from build123d import *

# Parameters (mm, degrees)
SKETCH1_W                = 60.014675034
SKETCH1_H                = 30.010951808
BOSS_EXTRUDE3_DEPTH      = 2
SKETCH5_R                = 0.958101179
SKETCH5_R_2              = 1
CUT_EXTRUDE2_DEPTH       = 2
BOSS_EXTRUDE5_DEPTH      = 10
BOSS_EXTRUDE5_DEPTH_BACK = 10


with BuildPart() as part:
    # Sketch1 → Boss-Extrude3 (new body)
    with BuildSketch(Plane(origin=(0, 0, 0), x_dir=(1, 0, 0), z_dir=(0, 1, 0))):
        Rectangle(SKETCH1_W, SKETCH1_H)
    extrude(amount=BOSS_EXTRUDE3_DEPTH)

    # Sketch5 → Cut-Extrude2 (cut)
    with BuildSketch(Plane(origin=(0, 2, 0), x_dir=(1, 0, 0), z_dir=(0, 1, 0))):
        with Locations(Location((28.355534017, 0, 0), (0, 0, 270))):
            Circle(SKETCH5_R)
        with Locations(Location((-28.355534017, 0, 0), (0, 0, 270))):
            Circle(SKETCH5_R_2)
    extrude(amount=-CUT_EXTRUDE2_DEPTH, mode=Mode.SUBTRACT)

    # Sketch7 → Boss-Extrude5 (add, two sides: drawn at the far end of the back side and taken through both)
    with BuildSketch(Plane.XY.offset(-BOSS_EXTRUDE5_DEPTH_BACK)):
        Polygon((7.498773608, 0), (8.961948947, 0), (8.961948947, -3.176146278), (21.045388571, -3.176146278), (21.045388571, 0), (22.508563909, 0), (22.508563909, -4.517390338), (7.498773608, -4.517390338), align=None)
        Polygon((-7.498773608, 0), (-7.498773608, -4.517390338), (-22.508563909, -4.517390338), (-22.508563909, 0), (-21.045388571, 0), (-21.045388571, -3.176146278), (-8.961948947, -3.176146278), (-8.961948947, 0), align=None)
    extrude(amount=BOSS_EXTRUDE5_DEPTH + BOSS_EXTRUDE5_DEPTH_BACK)


solid = part.part
Model file for the job. Use its own axes, mm. A direction names the side the tool comes from. Give positions to 0.01 mm unless a question says otherwise; leave off trailing zeros. Loops run counter-clockwise (first coordinate to the right, second up) from the corner with the lowest first, then second, coordinate; pieces in that order, holes last.
Item 1: Slice it at B-B (x = 17.5). Write the cut outline in (y, z), plus the area to 3 significant figures.
Check values:
outline: (-4.52, -10) - (-3.18, -10) - (-3.18, 10) - (-4.52, 10) - close; (0, -15.01) - (2, -15.01) - (2, 15.01) - (0, 15.01) - close
area: 86.8 mm2
Item 2: Drill centre lines: line 1 along X through (y, z) = (0.6, 0); line 2 along X through (y, z) = (-3, 2.5); line 3 along Y through (x, z) = (20, 5). Where is each one in solid material? Low to high.
Check values:
line 1: x = -30.01 to -29.36, -27.36 to 27.4, 29.31 to 30.01
line 2: x = -22.51 to -21.05, -8.96 to -7.5, 7.5 to 8.96, 21.05 to 22.51
line 3: y = -4.52 to -3.18, 0 to 2
Item 3: Slice it at D-D (z = -4). Write the cut outline in (x, y).
Check values:
outline: (-30.01, 0) - (-22.51, 0) - (-22.51, -4.52) - (-7.5, -4.52) - (-7.5, 0) - (7.5, 0) - (7.5, -4.52) - (22.51, -4.52) - (22.51, 0) - (30.01, 0) - (30.01, 2) - (-30.01, 2) - close; hole (-21.05, -3.18) - (-8.96, -3.18) - (-8.96, 0) - (-21.05, 0) - close; hole (8.96, -3.18) - (21.05, -3.18) - (21.05, 0) - (8.96, 0) - close
Item 4: Slice it at C-C (y = -1.25). Write the cut outline in (x, z), plus the area to 3 significant figures.
Check values:
outline: (-22.51, -10) - (-21.05, -10) - (-21.05, 10) - (-22.51, 10) - close; (-8.96, -10) - (-7.5, -10) - (-7.5, 10) - (-8.96, 10) - close; (7.5, -10) - (8.96, -10) - (8.96, 10) - (7.5, 10) - close; (21.05, -10) - (22.51, -10) - (22.51, 10) - (21.05, 10) - close
area: 117 mm2
Item 5: Which spindle directions (+Z, -Z, +X, -X, +Y, -Y) get a long thin tool onto all of the face, cutting with end or side? Do faces 1 (the face through (-15, -4, 10)), 2 (the face through (-22.509, -2, 0)), 3 (the face through (21.045, -2, 0)). Say none if no direction does.
Check values:
face 1: +Z, +X, -X, -Y
face 2: +Z, -Z, -X, -Y
face 3: +Z, -Z
Item 6: Slice it at A-A (z = 0). Write the cut outline in (x, y).
Check values:
outline: (-30.01, 0) - (-29.36, 0) - (-29.36, 2) - (-30.01, 2) - close; (-27.36, 0) - (-22.51, 0) - (-22.51, -4.52) - (-7.5, -4.52) - (-7.5, 0) - (7.5, 0) - (7.5, -4.52) - (22.51, -4.52) - (22.51, 0) - (27.4, 0) - (27.4, 2) - (-27.36, 2) - close; (29.31, 0) - (30.01, 0) - (30.01, 2) - (29.31, 2) - close; hole (-21.05, -3.18) - (-8.96, -3.18) - (-8.96, 0) - (-21.05, 0) - close; hole (8.96, -3.18) - (21.05, -3.18) - (21.05, 0) - (8.96, 0) - close
Item 7: Mould opens along Y. For faces 4 (the face through (0, 2, 0)), 5 (the face through (-8.962, -2, 0)), 6 (the face through (29.305, 1.014, -0.125)) say: +Y half, -Y half, draft (parallel to the pull), parting line (faces both ways), or undercut.
Check values:
face 4: +Y half
face 5: undercut
face 6: draft
Item 8: Drop flat-ended pins along their axis: P1, Ø3.5, axis at x = -18.5, y = -3, coming from the -Z side; P2, Ø1.5, axis at y = -3.5, z = -2, coming from the +X side; P3, Ø1.4, axis at y = -2, z = -4, coming from the -X side. Give the stop position or say it passes through.
Check values:
P1: stops at z = -10
P2: stops at x = 22.51
P3: stops at x = -22.51
